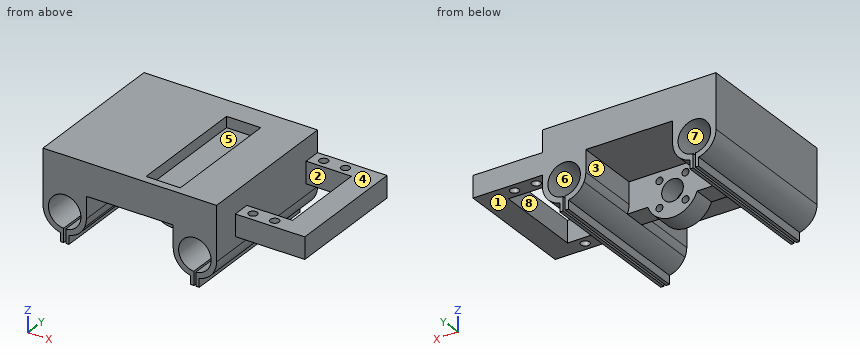
from build123d import *

# Parameters (mm, degrees)
SALIENTE_EXTRUIR1_DEPTH    = 70
SALIENTE_EXTRUIR2_START    = -70
SALIENTE_EXTRUIR2_DEPTH    = 70
CORTAR_EXTRUIR2_DEPTH      = 85.409715081
CORTAR_EXTRUIR2_DEPTH_BACK = 85.409715081
CORTAR_EXTRUIR3_START      = -30
CORTAR_EXTRUIR3_DEPTH      = 30
CORTAR_EXTRUIR6_DEPTH      = 30
CORTAR_EXTRUIR4_DEPTH      = 85.409715081
CORTAR_EXTRUIR4_DEPTH_BACK = 85.409715081
CROQUIS6_R                 = 5
CROQUIS6_R_2               = 1.6
CROQUIS7_W                 = 10
CROQUIS7_H                 = 8
SALIENTE_EXTRUIR3_DEPTH    = 32
CORTAR_EXTRUIR5_DEPTH      = 105.466848526
CORTAR_EXTRUIR5_DEPTH_BACK = 105.466848526
CROQUIS8_R                 = 2
SALIENTE_EXTRUIR4_REACH    = 100.25
CROQUIS10_W                = 11
CROQUIS10_H                = 10
CROQUIS12_W                = 15.8
CROQUIS12_H                = 55.8
CORTAR_EXTRUIR7_DEPTH      = 5


with BuildPart() as part:
    # Croquis1 → Saliente-Extruir1 (new body)
    with BuildSketch(Plane(origin=(0, 0, 0), x_dir=(1, 0, 0), z_dir=(0, 1, 0))):
        with BuildLine():
            Line((40, -25), (40, 0))
            ThreePointArc((40, 0), (32.043096437, 9.789063129), (20.83484861, 4))
            Line((20.83484861, 4), (11.313708499, 4))
            ThreePointArc((11.313708499, 4), (0, 12), (-11.313708499, 4))
            Line((-11.313708499, 4), (-20.83484861, 4))
            ThreePointArc((-20.83484861, 4), (-32.043096437, 9.789063129), (-40, 0))
            Line((-40, 0), (-40, -25))
            Line((-40, -25), (40, -25))
        make_face()
    extrude(amount=SALIENTE_EXTRUIR1_DEPTH)

    # Croquis3 → Saliente-Extruir2 (add)
    with BuildSketch(Plane(origin=(0, 70, 0), x_dir=(1, 0, 0), z_dir=(0, 1, 0)).offset(SALIENTE_EXTRUIR2_START)):
        with BuildLine():
            Line((-32, 9.797958971), (-32, 13.797958971))
            Line((-32, 13.797958971), (-28, 13.797958971))
            Line((-28, 13.797958971), (-28, 9.797958971))
            ThreePointArc((-28, 9.797958971), (-30, 10), (-32, 9.797958971))
        make_face()
        with BuildLine():
            Line((28, 9.797958971), (28, 13.797958971))
            Line((28, 13.797958971), (32, 13.797958971))
            Line((32, 13.797958971), (32, 9.797958971))
            ThreePointArc((32, 9.797958971), (30, 10), (28, 9.797958971))
        make_face()
    extrude(amount=SALIENTE_EXTRUIR2_DEPTH)

    # Croquis4 → Cortar-Extruir2 (cut, two sides: drawn at the far end of the back side and taken through both)
    with BuildSketch(Plane(origin=(0, 70, 0), x_dir=(1, 0, 0), z_dir=(0, 1, 0)).offset(-CORTAR_EXTRUIR2_DEPTH_BACK)):
        with BuildLine():
            Line((-30.5, 7.483314774), (-30.5, 14.654769407))
            Line((-30.5, 14.654769407), (-29.5, 14.654769407))
            Line((-29.5, 14.654769407), (-29.5, 7.483314774))
            ThreePointArc((-29.5, 7.483314774), (-30, -7.5), (-30.5, 7.483314774))
        make_face()
        with BuildLine():
            Line((29.5, 7.483314774), (29.5, 14.654769407))
            Line((29.5, 14.654769407), (30.5, 14.654769407))
            Line((30.5, 14.654769407), (30.5, 7.483314774))
            ThreePointArc((30.5, 7.483314774), (30, -7.5), (29.5, 7.483314774))
        make_face()
    extrude(amount=CORTAR_EXTRUIR2_DEPTH + CORTAR_EXTRUIR2_DEPTH_BACK, mode=Mode.SUBTRACT)

    # Croquis5 → Cortar-Extruir3 (cut)
    with BuildSketch(Plane(origin=(0, 70, 0), x_dir=(1, 0, 0), z_dir=(0, 1, 0)).offset(CORTAR_EXTRUIR3_START)):
        with BuildLine():
            Line((-20, 0), (-20, -10))
            Line((-20, -10), (20, -10))
            Line((20, -10), (20, 0))
            ThreePointArc((20, 0), (20.210936871, 2.043096437), (20.83484861, 4))
            Line((20.83484861, 4), (20.83484861, 13.99599321))
            Line((20.83484861, 13.99599321), (-20.83484861, 13.99599321))
            Line((-20.83484861, 13.99599321), (-20.83484861, 4))
            ThreePointArc((-20.83484861, 4), (-20.210936871, 2.043096437), (-20, 0))
        make_face()
    extrude(amount=CORTAR_EXTRUIR3_DEPTH, mode=Mode.SUBTRACT)

    # Croquis9 → Cortar-Extruir6 (cut)
    with BuildSketch(Plane(origin=(0, 0, 0), x_dir=(1, 0, 0), z_dir=(0, 1, 0))):
        with BuildLine():
            Line((-20, 0), (-20, -10))
            Line((-20, -10), (20, -10))
            Line((20, -10), (20, 0))
            ThreePointArc((20, 0), (20.210936871, 2.043096437), (20.83484861, 4))
            Line((20.83484861, 4), (20.83484861, 13.99599321))
            Line((20.83484861, 13.99599321), (-20.83484861, 13.99599321))
            Line((-20.83484861, 13.99599321), (-20.83484861, 4))
            ThreePointArc((-20.83484861, 4), (-20.210936871, 2.043096437), (-20, 0))
        make_face()
    extrude(amount=CORTAR_EXTRUIR6_DEPTH, mode=Mode.SUBTRACT)

    # Croquis6 → Cortar-Extruir4 (cut, two sides: drawn at the far end of the back side and taken through both)
    with BuildSketch(Plane(origin=(0, 70, 0), x_dir=(1, 0, 0), z_dir=(0, 1, 0)).offset(-CORTAR_EXTRUIR4_DEPTH_BACK)):
        with Locations(Location((0, 0, 0), (0, 0, 270))):
            Circle(CROQUIS6_R)
        with Locations(Location((-6.01040764, 6.01040764, 0), (0, 0, 270))):
            Circle(CROQUIS6_R_2)
        with Locations(Location((6.01040764, 6.01040764, 0), (0, 0, 270))):
            Circle(CROQUIS6_R_2)
        with Locations(Location((6.01040764, -6.01040764, 0), (0, 0, 270))):
            Circle(CROQUIS6_R_2)
        with Locations(Location((-6.01040764, -6.01040764, 0), (0, 0, 270))):
            Circle(CROQUIS6_R_2)
    extrude(amount=CORTAR_EXTRUIR4_DEPTH + CORTAR_EXTRUIR4_DEPTH_BACK, mode=Mode.SUBTRACT)

    # Croquis7 → Saliente-Extruir3 (add)
    with BuildSketch(Plane(origin=(40, 0, 0), x_dir=(0, 0, -1), z_dir=(1, 0, 0))):
        with Locations((-10, 66)):
            Rectangle(CROQUIS7_W, CROQUIS7_H)
        with Locations((-10, 17)):
            Rectangle(CROQUIS7_W, CROQUIS7_H)
    extrude(amount=SALIENTE_EXTRUIR3_DEPTH)

    # Croquis8 → Cortar-Extruir5 (cut, two sides: drawn at the far end of the back side and taken through both)
    with BuildSketch(Plane.XY.offset(15).offset(-CORTAR_EXTRUIR5_DEPTH_BACK)):
        with Locations((45.5, 66)):
            Circle(CROQUIS8_R)
        with Locations((55.5, 66)):
            Circle(CROQUIS8_R)
        with Locations((45.5, 17)):
            Circle(CROQUIS8_R)
        with Locations((55.5, 17)):
            Circle(CROQUIS8_R)
    extrude(amount=CORTAR_EXTRUIR5_DEPTH + CORTAR_EXTRUIR5_DEPTH_BACK, mode=Mode.SUBTRACT)

    # Croquis10 → Saliente-Extruir4 (add, up to next)
    with BuildSketch(Plane.XZ.offset(-62), mode=Mode.PRIVATE) as saliente_extruir4_sk1:
        with Locations((66.5, 10)):
            Rectangle(CROQUIS10_W, CROQUIS10_H)
    saliente_extruir4_tool1 = extrude(saliente_extruir4_sk1.sketch, amount=SALIENTE_EXTRUIR4_REACH, mode=Mode.PRIVATE) - part.part
    add(saliente_extruir4_tool1.solids().sort_by_distance((66.5, 62, 10))[0])

    # Croquis12 → Cortar-Extruir7 (cut)
    with BuildSketch(Plane.XY.offset(25)):
        with Locations((13, 31.5)):
            Rectangle(CROQUIS12_W, CROQUIS12_H)
    extrude(amount=-CORTAR_EXTRUIR7_DEPTH, mode=Mode.SUBTRACT)


solid = part.part
Input: part model. Units: mm. Frame: model coordinates. Face numbers are marked on the shaded views. A direction names the side the tool comes from. Give positions to 0.01 mm unless a question says otherwise; leave off trailing zeros. Order: outer loops, then holes, each group sorted by start corner. A loop starts at its lowest first (then second) coordinate and runs counter-clockwise, first axis right, second up. Notation, with made-up numbers: M -19,49 L -10,49 A11 cw -10,56 Z; hole C 88.5,75 d4. An arc over 180 degrees is marked long. Answer as a JSON object with one key per item and string values.
1. First-contact query: P1, Ø5.5, axis at x = 13.5, z = 22, coming from the -Y side; P2, Ø5, axis at y = 33.5, z = -10.5, coming from the -X side; P3, Ø5.5, axis at y = 25, z = 23, coming from the +X side; P4, Ø3, axis at x = 55.5, y = 66, coming from the +Z side. Flat tips, straight axial feed; report the tip coordinate or a pass-through.
Result sheet:
{"P1": "y = 0", "P2": "x = -36", "P3": "x = 40", "P4": "through"}
2. Cut plane C-C, the plane z = 13.5. Output: boundary loops of the cut face in (x, y), and give its area (3 significant figures).
Result sheet:
{"outline": "M -40,0 L 40,0 L 40,13 L 72,13 L 72,70 L -40,70 Z; hole M 40,21 L 61,21 L 61,62 L 40,62 Z; hole C 45.5,17 d4; hole C 45.5,66 d4; hole C 55.5,17 d4; hole C 55.5,66 d4", "area": "6,510 mm²"}
3. Ray query, line 1 (X direction, y = 59.5, z = -0.5); line 2 (X direction, y = 17, z = 11.5); line 3 (X direction, y = 50.5, z = 8). Return the intervals inside material, ascending. Write a range as [from, to].
Result sheet:
{"line 1": "[-39.99, -37.48], [-22.52, -20.01], [20.01, 22.52], [37.48, 39.99]", "line 2": "[-40, 43.5], [47.5, 53.5], [57.5, 72]", "line 3": "[-40, -20], [20, 40], [61, 72]"}
4. Pull-direction query (Z, two-part tool) for the marked faces 5, 6, 7 and 8; classes: +Z half, -Z half, draft (parallel to the pull), parting line (faces both ways), or undercut.
Result sheet:
{"face 5": "+Z half", "face 6": "undercut", "face 7": "undercut", "face 8": "draft"}
5. Cut plane D-D, the plane x = 0. Output: boundary loops of the cut face in (y, z), and give its area (3 significant figures).
Result sheet:
{"outline": "M 0,10 L 30,10 L 30,5 L 40,5 L 40,10 L 70,10 L 70,25 L 0,25 Z; M 30,-12 L 40,-12 L 40,-5 L 30,-5 Z", "area": "1,170 mm²"}
6. Cut plane A-A, the plane x = 55.5. Output: boundary loops of the cut face in (y, z), and give its area (3 significant figures).
Result sheet:
{"outline": "M 13,5 L 15,5 L 15,15 L 13,15 Z; M 19,5 L 21,5 L 21,15 L 19,15 Z; M 62,5 L 64,5 L 64,15 L 62,15 Z; M 68,5 L 70,5 L 70,15 L 68,15 Z", "area": "80.0 mm²"}
7. Reachability of the marked faces 1, 2, 3 and 4 from +Z, -Z, +X, -X, +Y, -Y: full face, straight path, thin tool, end or side. Return the list, or none.
Result sheet:
{"face 1": "-Z, +X, +Y, -Y", "face 2": "+Z, -Z", "face 3": "-Z, +Y", "face 4": "+Z, +X, +Y, -Y"}
